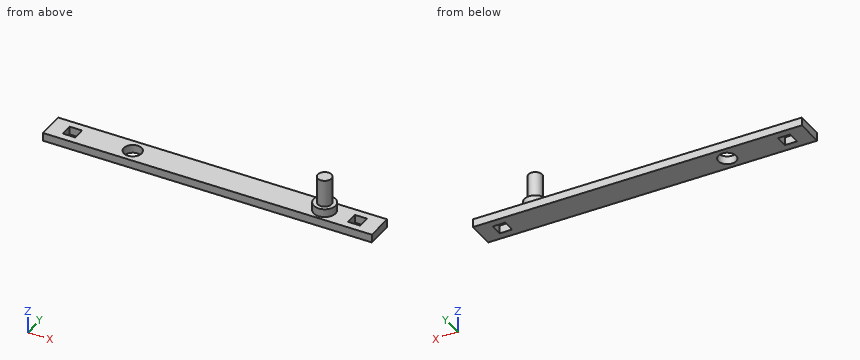
from build123d import *

# Parameters (mm, degrees)
F0_W     = 120
F0_H     = 10
F0_W_2   = 4.5
F0_H_2   = 4.5
F0_R     = 3.25
F1_DEPTH = 3
F2_R     = 4
F3_DEPTH = 3
F4_R     = 2.5
F5_DEPTH = 10


with BuildPart() as f1:
    # F0 (on Top) → F1 (new body)
    with BuildSketch(Plane.XY):
        Rectangle(F0_W, F0_H)
        with Locations((-52, 0)):
            Rectangle(F0_W_2, F0_H_2, mode=Mode.SUBTRACT)
        with Locations((-30, 0)):
            Circle(F0_R, mode=Mode.SUBTRACT)
        with Locations((52, 0)):
            Rectangle(F0_W_2, F0_H_2, mode=Mode.SUBTRACT)
    extrude(amount=F1_DEPTH)

    # F2 (on face) → F3 (join)
    with BuildSketch(Plane.XY.offset(3)):
        with Locations((40, 0)):
            Circle(F2_R)
    extrude(amount=F3_DEPTH)

    # F4 (on face) → F5 (join)
    with BuildSketch(Plane.XY.offset(6)):
        with Locations((40, 0)):
            Circle(F4_R)
    extrude(amount=F5_DEPTH)


solid = f1.part
Here's how the part is built. I have some questions about the finished solid (model axes, mm). Round coordinates to 2 decimals unless told otherwise and drop trailing zeros. Write each loop counter-clockwise with the first axis right and the second up, starting at its lowest first coordinate (ties: lowest second). Pieces come first, ordered by that corner, then holes. Notation, with made-up numbers: (85, 4) -> (117, 4) arc R23 cw to (117, 16) -> close; hole circle Ø7 at (-18.75, 11). An arc over 180 degrees is marked (long way). One line per item, written item: value.
1) I'm going to push flat-ended pins straight in: pin 1 Ø2 at (x, y) = (16, -3.5) entering from +Z; pin 2 Ø3 at (y, z) = (-0.5, 5) entering from +X. Where does each tip first touch, or does it pass through?
Filled sheet:
pin 1: stops at z = 3
pin 2: stops at x = 44
2) If I drill on line 1 (Y direction, x = -30, z = 1.65); line 2 (Z direction, x = 53, y = 2.75); line 3 (X direction, y = 0.75, z = 1.5), over which ranges is the centre line in solid material (lowest first)? Write a range as [from, to].
Filled sheet:
line 1: y = [-5, -3.25], [3.25, 5]
line 2: z = [0, 3]
line 3: x = [-60, -54.25], [-49.75, -33.16], [-26.84, 49.75], [54.25, 60]
3) Suppose I cut it at D-D on z = 14.75. List the corners of the cut face in (x, y) for me, plus the area to 3 significant figures.
Filled sheet:
outline: circle Ø5 at (40, 0)
area: 19.6 mm2
4) Suppose I cut it at C-C on x = 40. List the corners of the cut face in (y, z) for me, plus the area to 3 significant figures.
Filled sheet:
outline: (-5, 0) -> (5, 0) -> (5, 3) -> (4, 3) -> (4, 6) -> (2.5, 6) -> (2.5, 16) -> (-2.5, 16) -> (-2.5, 6) -> (-4, 6) -> (-4, 3) -> (-5, 3) -> close
area: 104 mm2
5) Suppose I cut it at A-A on x = -30. List the corners of the cut face in (y, z) for me, plus the area to 3 significant figures.
Filled sheet:
outline: (-5, 0) -> (-3.25, 0) -> (-3.25, 3) -> (-5, 3) -> close; (3.25, 0) -> (5, 0) -> (5, 3) -> (3.25, 3) -> close
area: 10.5 mm2
6) Suppose I cut it at B-B on z = 2. List the corners of the cut face in (x, y) for me, plus the area to 3 significant figures.
Filled sheet:
outline: (-60, -5) -> (60, -5) -> (60, 5) -> (-60, 5) -> close; hole (-54.25, -2.25) -> (-49.75, -2.25) -> (-49.75, 2.25) -> (-54.25, 2.25) -> close; hole circle Ø6.5 at (-30, 0); hole (49.75, -2.25) -> (54.25, -2.25) -> (54.25, 2.25) -> (49.75, 2.25) -> close
area: 1,130 mm2
